CAD build for the part. Positions are in the model's coordinates, mm. A direction names the side the tool comes from. Give positions to 0.01 mm unless a question says otherwise; leave off trailing zeros. Write each loop counter-clockwise with the first axis right and the second up, starting at its lowest first coordinate (ties: lowest second). Pieces come first, ordered by that corner, then holes. Notation, with made-up numbers: (-14, 30) - (19, 30) arc R6 cw to (19, 39) - close; hole circle Ø1 at (71, 71.25). An arc over 180 degrees is marked (long way). Put each result on its own line as item: value. Start each with the question number.
1. Mould opens along X. For faces 1 (the cylindrical face through (68.37, 0.07, 0.79)), 2 (the cylindrical face through (43.497, -51.897, 0.789)), 3 (the flat face through (52, -30, 1.6)) say: +X half, -X half, draft (parallel to the pull), parting line (faces both ways), or undercut.
2. Cut at C-C on x = 25. List the corners of the cut face in (y, z).
3. Cut at A-A on y = -23. List the corners of the cut face in (x, z).
4. Cut at B-B on x = 0. List the corners of the cut face in (y, z), and give its area (3 significant figures).
5. Tool access for faces 4 (the cylindrical face through (10.296, -50.46, 0.789)), 5 (the flat face through (34, 5, 1)): list every direction of +Z, -Z, +X, -X, +Y, -Y with a clear straight run to the whole face (end or side of a thin tool).
6. Cut at D-D on z = 0.85. Give the number of separate pieces and of enclosed holes in the cut face, and give its area (3 significant figures).
7. Wall check: line 1 (Y direction, x = 55, z = 0.75); line 2 (Y direction, x = 26, z = 0.7); line 3 (X direction, y = -18.5, z = 0.9). Give the ranges that are in metal, low to high.
from build123d import *

# Parameters (mm, degrees)
SKETCH1_W           = 80
SKETCH1_H           = 70
SKETCH1_R           = 1.63195
SKETCH1_R_2         = 1.1
BOSS_EXTRUDE1_DEPTH = 1.6


with BuildPart() as part:
    # Sketch1 → Boss-Extrude1 (new body)
    with BuildSketch(Plane.XY):
        with Locations((35, -30)):
            Rectangle(SKETCH1_W, SKETCH1_H)
        with Locations((0, -60)):
            Circle(SKETCH1_R, mode=Mode.SUBTRACT)
        with BuildLine():
            Line((7.7, -49.36805), (7.7, -13.63195))
            ThreePointArc((7.7, -13.63195), (10.268176474, -12.568176474), (11.33195, -10))
            Line((11.33195, -10), (41.06805, -10))
            ThreePointArc((41.06805, -10), (42.131823526, -12.568176474), (44.7, -13.63195))
            Line((44.7, -13.63195), (44.7, -49.36805))
            ThreePointArc((44.7, -49.36805), (42.131823526, -50.431823526), (41.06805, -53))
            Line((41.06805, -53), (11.33195, -53))
            ThreePointArc((11.33195, -53), (10.268176474, -50.431823526), (7.7, -49.36805))
        make_face(mode=Mode.SUBTRACT)
        with Locations((70, -60)):
            Circle(SKETCH1_R, mode=Mode.SUBTRACT)
        with Locations((55.2, -47)):
            Circle(SKETCH1_R_2, mode=Mode.SUBTRACT)
        with Locations((68.2, -47)):
            Circle(SKETCH1_R_2, mode=Mode.SUBTRACT)
        Circle(SKETCH1_R, mode=Mode.SUBTRACT)
        with Locations((55.2, -14)):
            Circle(SKETCH1_R_2, mode=Mode.SUBTRACT)
        with Locations((68.2, -14)):
            Circle(SKETCH1_R_2, mode=Mode.SUBTRACT)
        with Locations((70, 0)):
            Circle(SKETCH1_R, mode=Mode.SUBTRACT)
        with Locations((7.7, -10)):
            Circle(SKETCH1_R, mode=Mode.SUBTRACT)
        with Locations((44.7, -10)):
            Circle(SKETCH1_R, mode=Mode.SUBTRACT)
        with Locations((7.7, -53)):
            Circle(SKETCH1_R, mode=Mode.SUBTRACT)
        with Locations((44.7, -53)):
            Circle(SKETCH1_R, mode=Mode.SUBTRACT)
    extrude(amount=BOSS_EXTRUDE1_DEPTH)


solid = part.part
Report:
1. face 1: undercut
1. face 2: undercut
1. face 3: draft
2. outline: (-65, 0) - (-53, 0) - (-53, 1.6) - (-65, 1.6) - close; (-10, 0) - (5, 0) - (5, 1.6) - (-10, 1.6) - close
3. outline: (-5, 0) - (7.7, 0) - (7.7, 1.6) - (-5, 1.6) - close; (44.7, 0) - (75, 0) - (75, 1.6) - (44.7, 1.6) - close
4. outline: (-65, 0) - (-61.63, 0) - (-61.63, 1.6) - (-65, 1.6) - close; (-58.37, 0) - (-1.63, 0) - (-1.63, 1.6) - (-58.37, 1.6) - close; (1.63, 0) - (5, 0) - (5, 1.6) - (1.63, 1.6) - close
4. area: 102 mm²
5. face 4: +Z, -Z
5. face 5: +Z, -Z, +X, -X, +Y
6. separate pieces: 1
6. enclosed holes: 13
6. area: 3,970 mm²
7. line 1: y = -65 to -48.08, -45.92 to -15.08, -12.92 to 5
7. line 2: y = -65 to -53, -10 to 5
7. line 3: x = -5 to 7.7, 44.7 to 75
